from build123d import *

# Parameters (mm, degrees)
SKETCH2_W           = 50.8
SKETCH2_H           = 83.82
BOSS_EXTRUDE1_DEPTH = 3.175
SKETCH3_R           = 2.4892
CUT_EXTRUDE1_DEPTH  = 99.063821183
FILLET1_R           = 6.35


with BuildPart() as part:
    # Sketch2 → Boss-Extrude1 (new body)
    with BuildSketch(Plane.XY):
        with Locations((25.4, 41.91)):
            Rectangle(SKETCH2_W, SKETCH2_H)
    extrude(amount=-BOSS_EXTRUDE1_DEPTH)

    # Sketch3 → Cut-Extrude1 (cut, through all)
    with BuildSketch(Plane.XY):
        with Locations((12.7, 71.12)):
            Circle(SKETCH3_R)
        with Locations((38.1, 71.12)):
            Circle(SKETCH3_R)
        with Locations((12.7, 38.1)):
            Circle(SKETCH3_R)
        with Locations((12.7, 12.7)):
            Circle(SKETCH3_R)
        with Locations((12.7, -12.7)):
            Circle(SKETCH3_R)
        with Locations((12.7, -38.1)):
            Circle(SKETCH3_R)
        with Locations((12.7, -63.5)):
            Circle(SKETCH3_R)
        with Locations((38.1, 12.7)):
            Circle(SKETCH3_R)
        with Locations((38.1, -12.7)):
            Circle(SKETCH3_R)
        with Locations((38.1, -38.1)):
            Circle(SKETCH3_R)
        with Locations((38.1, -63.5)):
            Circle(SKETCH3_R)
        with Locations((38.1, 38.1)):
            Circle(SKETCH3_R)
    extrude(amount=-CUT_EXTRUDE1_DEPTH, mode=Mode.SUBTRACT)

    # Fillet1
    fillet1_edges = [part.edges().sort_by_distance(p)[0] for p in [
        (0, 83.82, -1.5875),
        (50.8, 83.82, -1.5875),
        (50.8, 0, -1.5875),
        (0, 0, -1.5875),
    ]]
    fillet(fillet1_edges, radius=FILLET1_R)


solid = part.part
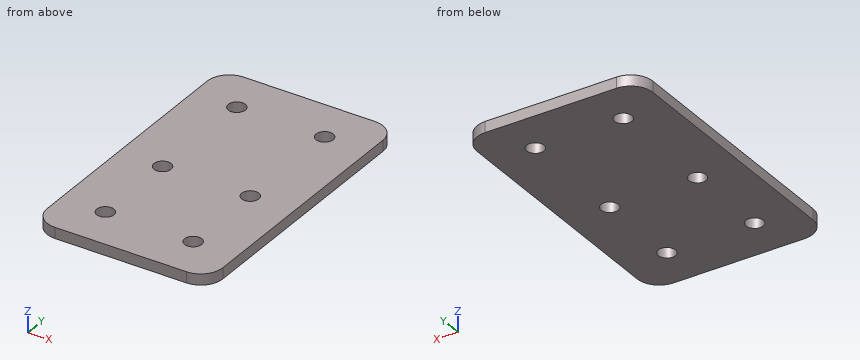
Check sheet for the modelled part. Datum: model origin and axes. Units: mm. Give positions to 0.01 mm unless a question says otherwise; leave off trailing zeros. Write each loop counter-clockwise with the first axis right and the second up, starting at its lowest first coordinate (ties: lowest second). Pieces come first, ordered by that corner, then holes. Notation, with made-up numbers: (4, 35.5) -> (32, 35.5) arc R23 cw to (32, 68.5) -> close; hole circle Ø2 at (-5, -12). An arc over 180 degrees is marked (long way). One line per item, written item: value. Start each with the question number.
Item 1: Section check A-A on x = 12.7. Record the cut outline in (y, z) (3 decimals), then the cut area to 3 significant figures.
Item 2: Section check B-B on z = -0.65. Record the cut outline in (x, y).
Item 3: Material ranges on probe 1 along Y at (x, z) = (12.7, -1.7); probe 2 along Y at (x, z) = (36.5, -2.3); probe 3 along X at (y, z) = (70, -0.4), recorded low to high. Write a range as from..to.
Item 4: Section check C-C on y = 71.12. Record the cut outline in (x, z) (3 decimals).
Item 5: Section check D-D on x = 37. Record the cut outline in (y, z) (3 decimals).
Results list:
1. outline: (0, -3.175) -> (10.211, -3.175) -> (10.211, 0) -> (0, 0) -> close; (15.189, -3.175) -> (35.611, -3.175) -> (35.611, 0) -> (15.189, 0) -> close; (40.589, -3.175) -> (68.631, -3.175) -> (68.631, 0) -> (40.589, 0) -> close; (73.609, -3.175) -> (83.82, -3.175) -> (83.82, 0) -> (73.609, 0) -> close
1. area: 219 mm²
2. outline: (0, 6.35) arc R6.35 ccw to (6.35, 0) -> (44.45, 0) arc R6.35 ccw to (50.8, 6.35) -> (50.8, 77.47) arc R6.35 ccw to (44.45, 83.82) -> (6.35, 83.82) arc R6.35 ccw to (0, 77.47) -> close; hole circle Ø4.98 at (12.7, 12.7); hole circle Ø4.98 at (12.7, 38.1); hole circle Ø4.98 at (12.7, 71.12); hole circle Ø4.98 at (38.1, 12.7); hole circle Ø4.98 at (38.1, 38.1); hole circle Ø4.98 at (38.1, 71.12)
3. probe 1: 0..10.21, 15.19..35.61, 40.59..68.63, 73.61..83.82
3. probe 2: 0..10.79, 14.61..36.19, 40.01..69.21, 73.03..83.82
3. probe 3: 0..10.48, 14.92..35.88, 40.32..50.8
4. outline: (0, -3.175) -> (10.211, -3.175) -> (10.211, 0) -> (0, 0) -> close; (15.189, -3.175) -> (35.611, -3.175) -> (35.611, 0) -> (15.189, 0) -> close; (40.589, -3.175) -> (50.8, -3.175) -> (50.8, 0) -> (40.589, 0) -> close
5. outline: (0, -3.175) -> (10.467, -3.175) -> (10.467, 0) -> (0, 0) -> close; (14.933, -3.175) -> (35.867, -3.175) -> (35.867, 0) -> (14.933, 0) -> close; (40.333, -3.175) -> (68.887, -3.175) -> (68.887, 0) -> (40.333, 0) -> close; (73.353, -3.175) -> (83.82, -3.175) -> (83.82, 0) -> (73.353, 0) -> close
